Here's how the part is built. I have some questions about the finished solid (model axes, mm). A direction names the side the tool comes from. Coordinates: 2 decimals unless noted, no trailing zeros. Write each loop counter-clockwise with the first axis right and the second up, starting at its lowest first coordinate (ties: lowest second). Pieces come first, ordered by that corner, then holes.
```python
from build123d import *

# Parameters (mm, degrees)
SKETCH1_R           = 7.9375
SKETCH1_R_2         = 14.2875
SKETCH1_R_3         = 3.429
BOSS_EXTRUDE1_DEPTH = 3.175


with BuildPart() as part:
    # Sketch1 → Boss-Extrude1 (new body)
    with BuildSketch(Plane(origin=(0, 0, 0), x_dir=(0, 0, -1), z_dir=(1, 0, 0))):
        with BuildLine():
            Line((25.4, 139.7), (25.4, 0))
            ThreePointArc((25.4, 0), (-11.359225326, -22.718450651), (-15.24, 20.32))
            ThreePointArc((-15.24, 20.32), (-13.370387337, 22.560193669), (-12.7, 25.4))
            Line((-12.7, 25.4), (-12.7, 114.3))
            ThreePointArc((-12.7, 114.3), (-13.370387337, 117.139806331), (-15.24, 119.38))
            ThreePointArc((-15.24, 119.38), (-11.359225326, 162.418450651), (25.4, 139.7))
        make_face()
        Circle(SKETCH1_R, mode=Mode.SUBTRACT)
        with Locations((0, 139.7)):
            Circle(SKETCH1_R_2, mode=Mode.SUBTRACT)
        with Locations((0, 15.875)):
            Circle(SKETCH1_R_3, mode=Mode.SUBTRACT)
        with Locations((15.875, 0)):
            Circle(SKETCH1_R_3, mode=Mode.SUBTRACT)
        with Locations((0, -15.875)):
            Circle(SKETCH1_R_3, mode=Mode.SUBTRACT)
        with Locations((-15.875, 0)):
            Circle(SKETCH1_R_3, mode=Mode.SUBTRACT)
    extrude(amount=BOSS_EXTRUDE1_DEPTH)


solid = part.part
```
1) Imagine slicing it at C-C on y = 134.5. Please give me the cut outline in (x, z) (3 decimals).
Values follow:
outline: (0, -25.4) - (3.175, -25.4) - (3.175, -13.308) - (0, -13.308) - close; (0, 13.308) - (3.175, 13.308) - (3.175, 24.862) - (0, 24.862) - close
2) Imagine slicing it at D-D on x = 1.8. Count the separate pieces of the cut face and the enclosed holes in it, then the cut area to 3 significant figures.
Values follow:
separate pieces: 1
enclosed holes: 6
area: 6,760 mm2
3) We'd pull the mould along Z, two halves only. Please class faces 3 (the face through (2, 69, 12.7)), 4 (the face through (1.57, -12.98, -1.84)), 5 (the face through (1.565, 19.275, 0.446)), 6 (the face through (3.175, 71, -6)): pulls with the +Z half, pulls with the -Z half, needs draft (parallel to the pull), parting line crosses it, or undercut.
Values follow:
face 3: pulls with the +Z half
face 4: undercut
face 5: undercut
face 6: needs draft
4) Imagine slicing it at B-B on z = 21. Please give me the cut outline in (x, y) (3 decimals).
Values follow:
outline: (0, -14.288) - (3.175, -14.288) - (3.175, 14.288) - (0, 14.288) - close; (0, 125.412) - (3.175, 125.412) - (3.175, 153.988) - (0, 153.988) - close
5) On a 3-axis mill with a long thin cutter (end or side, diameter ignored), from which of +Z, -Z, +X, -X, +Y, -Y can I reach the whole of each face in a straight line? I mean faces 1 (the face through (1.6, 22.5, 13.4)), 2 (the face through (0, 71, -6)). Say none if no direction works.
Values follow:
face 1: +Z, +X, -X
face 2: +Z, -Z, -X, +Y, -Y
6) Will these pins go through, and if not, where does the flat tip stop? pin 1 (1 mm diameter, centred on x = 0.5, z = 0.5, fed in from -Y); pin 2 (1.5 mm diameter, centred on x = 0.5, z = 12.5, fed in from +Y).
Values follow:
pin 1: stops at y = -25.4
pin 2: stops at y = 162.22
7) I need wall thicknesses on probe 1 along Y at (x, z) = (2.2, 0); probe 2 along Z at (x, y) = (2.85, 1); probe 3 along Y at (x, z) = (0.55, -7). Which ranges of each line are inside material? Lowest first, please.
Values follow:
probe 1: y = -25.4 to -19.3, -12.45 to -7.94, 7.94 to 12.45, 19.3 to 125.41, 153.99 to 165.1
probe 2: z = -25.4 to -19.15, -12.6 to -7.87, 7.87 to 12.6, 19.15 to 25.38
probe 3: y = -24.42 to -3.74, 3.74 to 127.24, 152.16 to 164.12
8) Imagine slicing it at A-A on z = 0. Please give me the cut outline in (x, y) (1 decimal), then the cut area to 3 significant figures.
Values follow:
outline: (0, -25.4) - (3.2, -25.4) - (3.2, -19.3) - (0, -19.3) - close; (0, -12.4) - (3.2, -12.4) - (3.2, -7.9) - (0, -7.9) - close; (0, 7.9) - (3.2, 7.9) - (3.2, 12.4) - (0, 12.4) - close; (0, 19.3) - (3.2, 19.3) - (3.2, 125.4) - (0, 125.4) - close; (0, 154) - (3.2, 154) - (3.2, 165.1) - (0, 165.1) - close
area: 420 mm2
